For this review, use the dimensioned drawing (mm, ordinates from the lowest corner) and the shaded views. A direction names the side the tool comes from. Give positions to 0.01 mm unless a question says otherwise; leave off trailing zeros. Write each loop counter-clockwise with the first axis right and the second up, starting at its lowest first coordinate (ties: lowest second). Pieces come first, ordered by that corner, then holes. Notation, with made-up numbers: (33, 7.25) - (39, 7.25) arc R16 ccw to (39, 38.25) - close; hole circle Ø8 at (-14, 84.5). An arc over 180 degrees is marked (long way). Use a Markdown table: item, result. Add a question column.
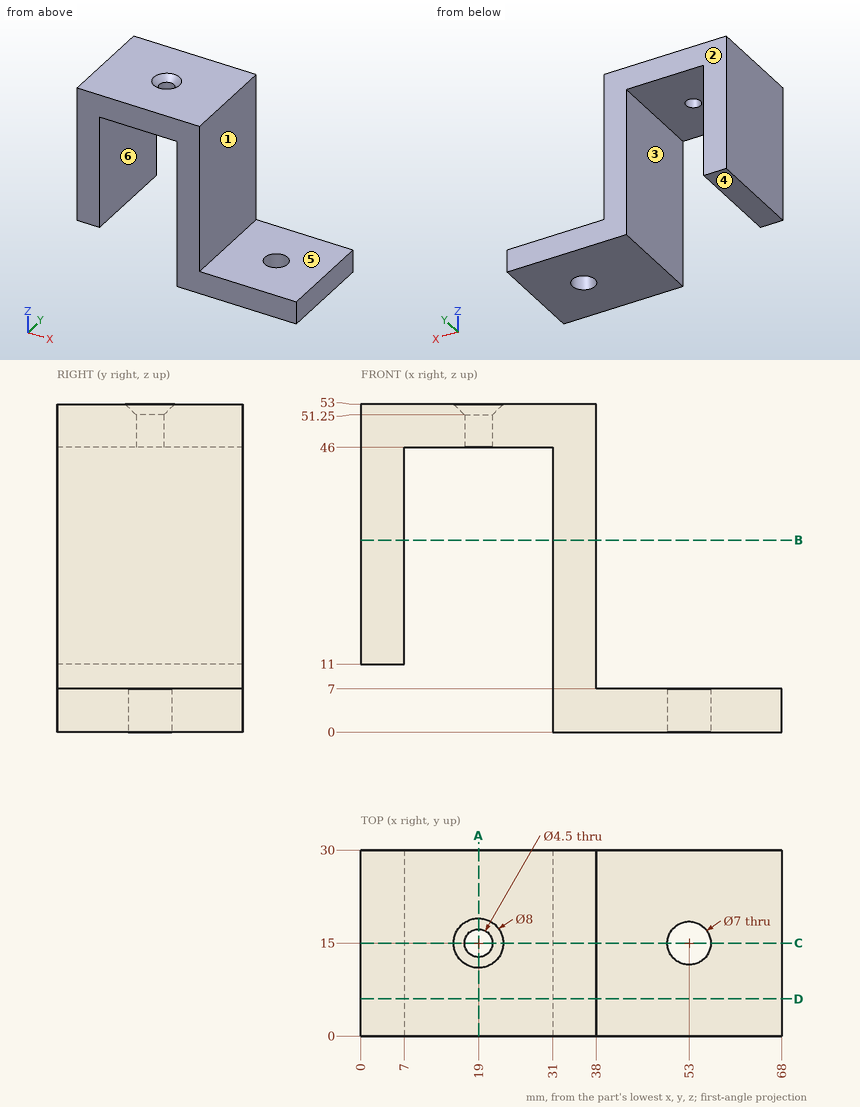
(1) For line 1 along Y through (x, z) = (19, 48); line 2 along X through (y, z) = (7, 36); line 3 along Z through (x, y) = (53, 27.5), list the stretches that pass through material, from the lowest coordinate up.
(2) Insertion check: pin 1 (6 mm diameter, centred on x = 29.5, z = 5.5, fed in from +Y); pin 2 (5 mm diameter, centred on x = 19, y = 15, fed in from -Z); pin 3 (15 mm diameter, centred on x = 53, y = 10.5, fed in from +Z); pin 4 (6 mm diameter, centred on y = 10.5, z = 25.5, fed in from +X). Each pin has a flat end and moves straight along its axis. Give the tip position at first contact, or say it passes through.
(3) Add section C-C (y = 15). State the section outline as (x, z) points.
(4) Tool access review of the marked faces 4, 5 and 6: name each direction out of +Z, -Z, +X, -X, +Y, -Y from which nothing blocks a thin tool from reaching the whole face with its end or side.
(5) Add section A-A (x = 19). State the section outline as (y, z) points, and give its area (3 significant figures).
(6) Add section D-D (y = 6). State the section outline as (x, z) points.
(7) Add section B-B (z = 31). State the section outline as (x, y) points, and give its area (3 significant figures).
(8) Mouldability with a two-part tool opening along X and no side actions: class the marked faces 1, 2 and 3 as +X half, -X half, draft (parallel to the pull), parting line (faces both ways), or undercut.
Answers follow:
| question | item | result |
|---|---|---|
| 1 | line 1 | 0 to 12.75, 17.25 to 30 |
| 1 | line 2 | 0 to 7, 31 to 38 |
| 1 | line 3 | 0 to 7 |
| 2 | pin 1 | y = 30 |
| 2 | pin 2 | z = 46 |
| 2 | pin 3 | z = 7 |
| 2 | pin 4 | x = 38 |
| 3 | outline | (0, 11) - (7, 11) - (7, 46) - (16.75, 46) - (16.75, 51.25) - (15, 53) - (0, 53) - close; (21.25, 46) - (31, 46) - (31, 0) - (49.5, 0) - (49.5, 7) - (38, 7) - (38, 53) - (23, 53) - (21.25, 51.25) - close; (56.5, 0) - (68, 0) - (68, 7) - (56.5, 7) - close |
| 4 | face 4 | -Z, -X, +Y, -Y |
| 4 | face 5 | +Z, +X, +Y, -Y |
| 4 | face 6 | -Z, +Y, -Y |
| 5 | outline | (0, 46) - (12.75, 46) - (12.75, 51.25) - (11, 53) - (0, 53) - close; (17.25, 46) - (30, 46) - (30, 53) - (19, 53) - (17.25, 51.25) - close |
| 5 | area | 175 mm^2 |
| 6 | outline | (0, 11) - (7, 11) - (7, 46) - (31, 46) - (31, 0) - (68, 0) - (68, 7) - (38, 7) - (38, 53) - (0, 53) - close |
| 7 | outline | (0, 0) - (7, 0) - (7, 30) - (0, 30) - close; (31, 0) - (38, 0) - (38, 30) - (31, 30) - close |
| 7 | area | 420 mm^2 |
| 8 | face 1 | +X half |
| 8 | face 2 | draft |
| 8 | face 3 | undercut |
